Can you work these out from the model? Positions are in its coordinate system, mm. A direction names the side the tool comes from. Round coordinates to 2 decimals unless told otherwise and drop trailing zeros. Order: outer loops, then holes, each group sorted by start corner. A loop starts at its lowest first (then second) coordinate and runs counter-clockwise, first axis right, second up. Notation, with made-up numbers: M -37.75,3 L 11.25,3 A20 ccw 11.25,28 Z; hole C -5.75,11 d5. An arc over 180 degrees is marked long. Answer as a JSON object with one key per item and string values. Group by question number.
Autodesk Inventor part; units mm, degrees
ref_plane "YZ Plane" through (0, 0, 0) normal (1, 0, 0) x (0, 1, 0)
ref_plane "XZ Plane" through (0, 0, 0) normal (0, 1, 0) x (-1, 0, 0)
ref_plane "XY Plane" through (0, 0, 0) normal (0, 0, 1) x (1, 0, 0)
sketch "Sketch1" plane through (0, 0, 0) normal (0, 0, 1) x (1, 0, 0)
  line L0 (0, 0) -> (36, 0)
  line L1 (36, 0) -> (36, 12)
  line L2 (36, 12) -> (24, 12)
  line L3 (24, 12) -> (24, 22)
  line L4 (24, 22) -> (12, 22)
  line L5 (12, 22) -> (12, 12)
  line L6 (12, 12) -> (0, 12)
  line L7 (0, 12) -> (0, 0)
  dimension "d0" = 36
  dimension "d1" = 12
  dimension "d2" = 12
  dimension "d3" = 10
  dimension "d4" = 12
extrude "Extrusion1" add sketch "Sketch1" along normal blind 108
sketch "Sketch2" plane through (0, 0, 0) normal (0, -1, 0) x (1, 0, 0)
  circle A0 centre (18, 4.5) radius 1.725
  line L0 (0, 0) -> (36, 0)
  line L1 (36, 0) -> (36, 108)
  circle A1 centre (18, 103.5) radius 1.725
  line L2 (0, 108) -> (36, 108)
  dimension "d7" = 3.45
  dimension "d8" = 4.5
  dimension "d9" = 18
  dimension "d10" = 3.45
  dimension "d11" = 18
  dimension "d12" = 4.5
extrude "Extrusion2" cut sketch "Sketch2" against normal blind 20
sketch "Sketch3" plane through (12, 22, 0) normal (0, 1, 0) x (1, 0, 0)
  circle A0 centre (6, -4.5) radius 1.725
  circle A1 centre (6, -4.5) radius 3
  circle A2 centre (6, -103.5) radius 1.725
  circle A3 centre (6, -103.5) radius 3
  point P0 (-12, 0)
  dimension "d15" = 6
  dimension "d16" = 6
extrude "Extrusion3" cut sketch "Sketch3" against normal blind 2 contours A0 | A1 | A2 | A3
sketch "Sketch4" plane through (36, 0, 0) normal (1, 0, 0) x (0, 0, -1)
  line L0 (-108, 0) -> (-107.85, 0)
  line L1 (0, 0) -> (-108, 0)
  line L2 (-107.85, 0) -> (-107.85, 12)
  line L3 (0, 12) -> (-108, 12)
  line L4 (-108, 0) -> (-108, 12)
  line L5 (-108, 12) -> (-108, 0)
  line L6 (-108, 22) -> (-107.85, 22)
  line L7 (-107.85, 12) -> (-108, 12)
  line L8 (0, 0) -> (-0.15, 0)
  line L9 (-0.15, 0) -> (-0.15, 12)
  line L10 (-0.15, 12) -> (0, 12)
  line L11 (0, 12) -> (0, 0)
  line L12 (0, 22) -> (-0.15, 22)
  line L13 (-0.15, 12) -> (0, 12)
  dimension "d19" = 0.15
  dimension "d20" = 12
  dimension "d21" = 0.15
  dimension "d22" = 0.15
extrude "Extrusion4" cut sketch "Sketch4" against normal through all contours L4 L3 L2 L0 | L9 L3 L11 L1
sketch "Sketch5" plane through (24, 22, 108) normal (1, 0, 0) x (0, 0, -1)
  line L0 (108, -10) -> (108, 0)
  line L1 (108, 0) -> (0, 0)
  line L2 (108, -10) -> (107.85, -10)
  line L3 (107.85, -10) -> (107.85, 0)
  line L4 (107.85, 0) -> (108, 0)
  line L5 (108, 0) -> (108, -10)
  line L6 (0.15, -10) -> (0, -10)
  line L7 (0, -10) -> (0, 0)
  line L8 (0.15, -10) -> (0, -10)
  line L9 (0, -10) -> (0, 0)
  line L10 (0, 0) -> (0.15, 0)
  line L11 (0.15, 0) -> (0.15, -10)
  point P0 (108, -22)
  dimension "d25" = 0.15
extrude "Extrusion5" cut sketch "Sketch5" against normal through all
sketch "Sketch6" plane through (12, 22, 0.15) normal (0, 1, 0) x (1, 0, 0)
  line L0 (0, 0) -> (0, -107.7)
  line L1 (12, 0) -> (12, -107.7)
  line L2 (0, -98.85) -> (12, -98.85)
  line L3 (12, -98.85) -> (12, -8.85)
  line L4 (12, -8.85) -> (0, -8.85)
  line L5 (0, -8.85) -> (0, -98.85)
  point P0 (-12, 0.15)
  dimension "d28" = 8.85
  dimension "d29" = 8.85
sketch "Sketch7" plane through (0, 0, 107.85) normal (0, -1, 0) x (1, 0, 0)
  line L0 (0, -107.7) -> (36, -107.7)
  line L1 (11.85, -107.7) -> (24.15, -107.7)
  line L2 (24.15, -107.7) -> (24.15, -98.55)
  line L3 (24.15, -98.55) -> (11.85, -98.55)
  line L4 (11.85, -98.55) -> (11.85, -107.7)
  line L5 (0, 0) -> (12, 0)
  line L6 (11.85, 0) -> (24.15, 0)
  line L7 (24.15, 0) -> (24.15, -9.15)
  line L8 (24.15, -9.15) -> (11.85, -9.15)
  line L9 (11.85, -9.15) -> (11.85, 0)
  line L10 (36, -107.7) -> (36, 0)
  point P0 (0, -107.85)
  dimension "d30" = 11.85
  dimension "d31" = 11.85
  dimension "d32" = 9.15
  dimension "d33" = 11.85
  dimension "d34" = 11.85
  dimension "d35" = 9.15
extrude "Extrusion6" cut sketch "Sketch7" against normal blind 6
sketch "Sketch8" plane through (36, 0, 0.15) normal (0, -1, 0) x (1, 0, 0)
  line L0 (-21, 95.7) -> (-15, 95.7)
  line L1 (-15, 95.7) -> (-15, 12)
  line L2 (-15, 12) -> (-21, 12)
  line L3 (-21, 12) -> (-21, 95.7)
  line L4 (-11.85, 0) -> (-24.15, 0)
  line L5 (0, 107.7) -> (-11.85, 107.7)
  line L6 (-24, 0) -> (-24, 107.7)
  line L7 (-12, 0) -> (-12, 107.7)
  point P0 (-36, -0.15)
  dimension "d38" = 12
  dimension "d39" = 12
  dimension "d40" = 3
  dimension "d41" = 3
extrude "Extrusion7" cut sketch "Sketch8" against normal through all
sketch "Sketch9" plane through (24, 12, 107.85) normal (0, 1, 0) x (1, 0, 0)
  line L0 (9, 3) -> (0, 3)
  line L1 (0, 3) -> (0, 104.7)
  line L2 (0, 104.7) -> (9, 104.7)
  line L3 (9, 104.7) -> (9, 3)
  line L4 (-12, 3) -> (-21, 3)
  line L5 (-21, 3) -> (-21, 104.7)
  line L6 (-21, 104.7) -> (-12, 104.7)
  line L7 (-12, 104.7) -> (-12, 3)
  line L8 (12, 0) -> (0.15, 0)
  line L9 (12, 107.7) -> (0, 107.7)
  line L10 (12, 107.7) -> (12, 0)
  line L11 (-24, 107.7) -> (-24, 0)
  line L12 (-12, 107.7) -> (-24, 107.7)
  line L13 (-24, 0) -> (-12, 0)
  line L14 (-12, 107.7) -> (-12, 0)
  line L15 (0, 107.7) -> (0, 0)
  point P0 (-24, 107.85)
  dimension "d44" = 3
  dimension "d45" = 3
  dimension "d46" = 3
  dimension "d47" = 3
  dimension "d48" = 3
  dimension "d49" = 3
  dimension "d50" = 0
  dimension "d51" = 0
extrude "Extrusion8" cut sketch "Sketch9" against normal through all contours L0 L1 L2 L3 | L4 L5 L6 L7
sketch "Sketch10" plane through (12, 0, 98.7) normal (0, -1, 0) x (1, 0, 0)
  line L0 (3, -86.55) -> (3, -2.85)
  line L1 (9, -2.85) -> (9, -86.55)
  line L2 (3, -2.85) -> (9, -2.85)
  line L3 (9, -2.85) -> (9, -86.55)
  line L4 (9, -86.55) -> (3, -86.55)
  line L5 (3, -86.55) -> (3, -2.85)
  line L6 (0, 0) -> (0, -89.4)
  line L7 (12, -98.55) -> (12, 9.15)
  line L8 (0, 0) -> (12, 0)
  line L9 (12, 0) -> (12, -89.4)
  line L10 (12, -89.4) -> (0, -89.4)
  line L11 (0, -89.4) -> (0, 0)
  line L12 (12, -89.4) -> (0, -89.4)
  line L13 (0, -89.4) -> (0, 0)
  line L14 (0, 0) -> (12, 0)
  line L15 (12, 0) -> (12, -89.4)
  point P0 (-12, -98.7)
properties part number "centerbeam"
1) If we section it at B-B on x = 27.5: Write out the boundary of the cut face in (y, z), plus the area to 3 significant figures.
2) If we section it at A-A on z = 39: Write out the boundary of the cut face in (x, y), plus the area to 3 significant figures.
3) I need wall thicknesses on line 1 along Z through (x, y) = (18, 21.15); line 2 along X through (y, z) = (5, 39.5); line 3 along Z through (x, y) = (18, 11.5) (3 decimals). Which ranges of each line are inside material? Lowest first, please.
4) For pin 1 (3 mm diameter, centred on x = 18.5, z = 4, fed in from +Y); pin 2 (3 mm diameter, centred on x = 30, z = 90, fed in from +Y); pin 3 (4 mm diameter, centred on y = 17, z = 76.5, fed in from +X); pin 4 (4.5 mm diameter, centred on x = 20.5, z = 101.5, fed in from -Y), each with a flat end and sliding along its axis, tell me the tip position at first contact or that it passes through.
5) If we section it at D-D on y = 10: Write out the boundary of the cut face in (x, z) (3 decimals).
6) We'd pull the mould along X, two halves only. Please class faces 6 (the face through (15, 11, 53)), 7 (the face through (18, 11, 12.15)), 8 (the face through (18, 8, 107.85)), 9 (the face through (36, 6, 53)): +X half, -X half, draft (parallel to the pull), parting line (faces both ways), or undercut.
7) If we section it at C-C on y = 16: Write out the boundary of the cut face in (x, z) (3 decimals), plus the area to 3 significant figures.
8) Which directions (+Z, -Z, +X, -X, +Y, -Y) give clear straight access to the entire face, cutting with the end or side of a thin tool? Please do faces 1 (the face through (34, 12, 54)), 2 (the face through (2, 0, 54)), 3 (the face through (21, 11, 55)), 4 (the face through (2, 12, 54)), 5 (the face through (20, 20, 4)).
Findings:
{
 "1": {"outline": "M 0,0.15 L 12,0.15 L 12,3.15 L 0,3.15 Z; M 0,104.85 L 12,104.85 L 12,107.85 L 0,107.85 Z", "area": "72.0 mm^2"},
 "2": {"outline": "M 0,0 L 3,0 L 3,12 L 0,12 Z; M 12,0 L 15,0 L 15,22 L 12,22 Z; M 21,0 L 24,0 L 24,22 L 21,22 Z; M 33,0 L 36,0 L 36,12 L 33,12 Z", "area": "204 mm^2"},
 "3": {"line 1": "z = 0.15 to 1.5, 7.5 to 12.15, 95.85 to 100.5, 106.5 to 107.85", "line 2": "x = 0 to 3, 12 to 15, 21 to 24, 33 to 36", "line 3": "z = 0.15 to 2.775, 6.225 to 12.15, 95.85 to 101.775, 105.225 to 107.85"},
 "4": {"pin 1": "stops at y = 20", "pin 2": "passes through", "pin 3": "stops at x = 24", "pin 4": "stops at y = 6"},
 "5": {"outline": "M 0,0.15 L 36,0.15 L 36,107.85 L 0,107.85 Z; hole M 3,3.15 L 12,3.15 L 12,104.85 L 3,104.85 Z; hole M 15,12.15 L 21,12.15 L 21,95.85 L 15,95.85 Z; hole C 18,4.5 d3.45; hole C 18,103.5 d3.45; hole M 24,3.15 L 33,3.15 L 33,104.85 L 24,104.85 Z"},
 "6": {"face 6": "undercut", "face 7": "undercut", "face 8": "draft", "face 9": "+X half"},
 "7": {"outline": "M 12,0.15 L 24,0.15 L 24,107.85 L 12,107.85 Z; hole M 15,12.15 L 21,12.15 L 21,95.85 L 15,95.85 Z; hole C 18,4.5 d3.45; hole C 18,103.5 d3.45", "area": "772 mm^2"},
 "8": {"face 1": "+Z, -Z, +X, +Y", "face 2": "+Z, -Z, +X, -X, -Y", "face 3": "+Y, -Y", "face 4": "+Z, -Z, -X, +Y", "face 5": "+Y"}
}
